```python
from build123d import *

# Parameters (mm, degrees)
F1_R     = 7.5
F2_DEPTH = 30
F3_R     = 12.5
F4_DEPTH = 25
F5_R     = 11
F6_DEPTH = 18.1
F8_W     = 15
F8_H     = 30.954544
F9_DEPTH = 25


with BuildPart() as f2:
    # F1 (on Front) → F2 (new body)
    with BuildSketch(Plane.XZ):
        Circle(F1_R)
    extrude(amount=F2_DEPTH)

    # F3 (on offset) → F4 (join)
    with BuildSketch(Plane.YZ.offset(7.8)):
        Circle(F3_R)
    extrude(amount=-F4_DEPTH)

    # F5 (on face) → F6 (cut)
    with BuildSketch(Plane(origin=(-17.2, 0, 0), x_dir=(0, -1, 0), z_dir=(-1, 0, 0))):
        Circle(F5_R)
    extrude(amount=-F6_DEPTH, mode=Mode.SUBTRACT)

    # F8 (on offset) → F9 (cut)
    with BuildSketch(Plane.YZ.offset(-7.4)):
        with Locations((7.5, 0)):
            Rectangle(F8_W, F8_H)
    extrude(amount=-F9_DEPTH, mode=Mode.SUBTRACT)


solid = f2.part
```
The listing builds one solid part. Answer for the finished solid, in the listing's coordinates (mm). A direction names the side the tool comes from. Coordinates: 2 decimals unless noted, no trailing zeros. Loops run counter-clockwise (first coordinate to the right, second up) from the corner with the lowest first, then second, coordinate; pieces in that order, holes last. Notation, with made-up numbers: (-8, 40.25) - (33, 40.25) arc R18 cw to (33, 53.25) - close; hole circle Ø4 at (83, 42.5). An arc over 180 degrees is marked (long way). Write item = value, one per line.
1) Section A-A (z = 0) is taken. Determine the outline of the cut face in (x, y), plus the area to 3 significant figures.
Responses:
outline = (-17.2, -12.5) - (-7.5, -12.5) - (-7.5, -30) - (7.5, -30) - (7.5, -12.5) - (7.8, -12.5) - (7.8, 12.5) - (-7.4, 12.5) - (-7.4, 11) - (0.9, 11) - (0.9, -11) - (-17.2, -11) - close
area = 475 mm^2
2) Which of the six approach directions +Z, -Z, +X, -X, +Y, -Y give full straight-line access (tool end or side, diameter ignored) to faces 1 (the face through (-7.4, 11.3, 1)), 2 (the face through (6.93, -19.86, -2.87)), 3 (the face through (-6.266, -10.492, 3.304))?
Responses:
face_1 = +Z, -Z, -X, +Y
face_2 = -Y
face_3 = -X
3) Section B-B (x = 0) is taken. Determine the outline of the cut face in (y, z).
Responses:
outline = (-30, -7.5) - (-10, -7.5) arc R12.5 ccw (long way) to (-10, 7.5) - (-30, 7.5) - close; hole circle Ø22 at (0, 0)
4) Find the intervals of material crossed by line 1 along Y through (x, z) = (-2.75, 0); line 2 along Y through (x, z) = (-9.25, 0); line 3 along X through (y, z) = (-28, -0.25), in increasing order.
Responses:
line_1 = -30 to -11, 11 to 12.5
line_2 = -12.5 to -11
line_3 = -7.5 to 7.5
5) Determine the mould class of faces 4 (the face through (0.9, 0, 0)), 5 (the face through (-12, 0, -12)), 6 (the face through (0, -30, 0)) for opening direction Y: pulls with the +Y half, pulls with the -Y half, needs draft (parallel to the pull), parting line crosses it, or undercut.
Responses:
face_4 = undercut
face_5 = pulls with the +Y half
face_6 = pulls with the -Y half
6) Each of these flat-tipped pins is pushed along its axis until it touches: P1, Ø3, axis at y = -23, z = 3.5, coming from the +X side; P2, Ø1.6, axis at x = -10.5, z = 12, coming from the +Y side; P3, Ø8, axis at x = -8.5, z = 5.5, coming from the -Y side; P4, Ø4, axis at x = 2.5, z = 6.5, coming from the +Y side. Where does it stop, or does it pass through?
Responses:
P1 = 7.23
P2 = 0
P3 = -30
P4 = 11.66
7) Section C-C (y = -6.5) is taken. Determine the outline of the cut face in (x, z).
Responses:
outline = (-17.2, -10.68) - (7.8, -10.68) - (7.8, 10.68) - (-17.2, 10.68) - (-17.2, 8.87) - (0.9, 8.87) - (0.9, -8.87) - (-17.2, -8.87) - close
8) Section D-D (z = -4.5) is taken. Determine the outline of the cut face in (x, y), plus the area to 3 significant figures.
Responses:
outline = (-17.2, -11.66) - (-6, -11.66) - (-6, -30) - (6, -30) - (6, -11.66) - (7.8, -11.66) - (7.8, 11.66) - (-7.4, 11.66) - (-7.4, 10.04) - (0.9, 10.04) - (0.9, -10.04) - (-17.2, -10.04) - close
area = 424 mm^2
